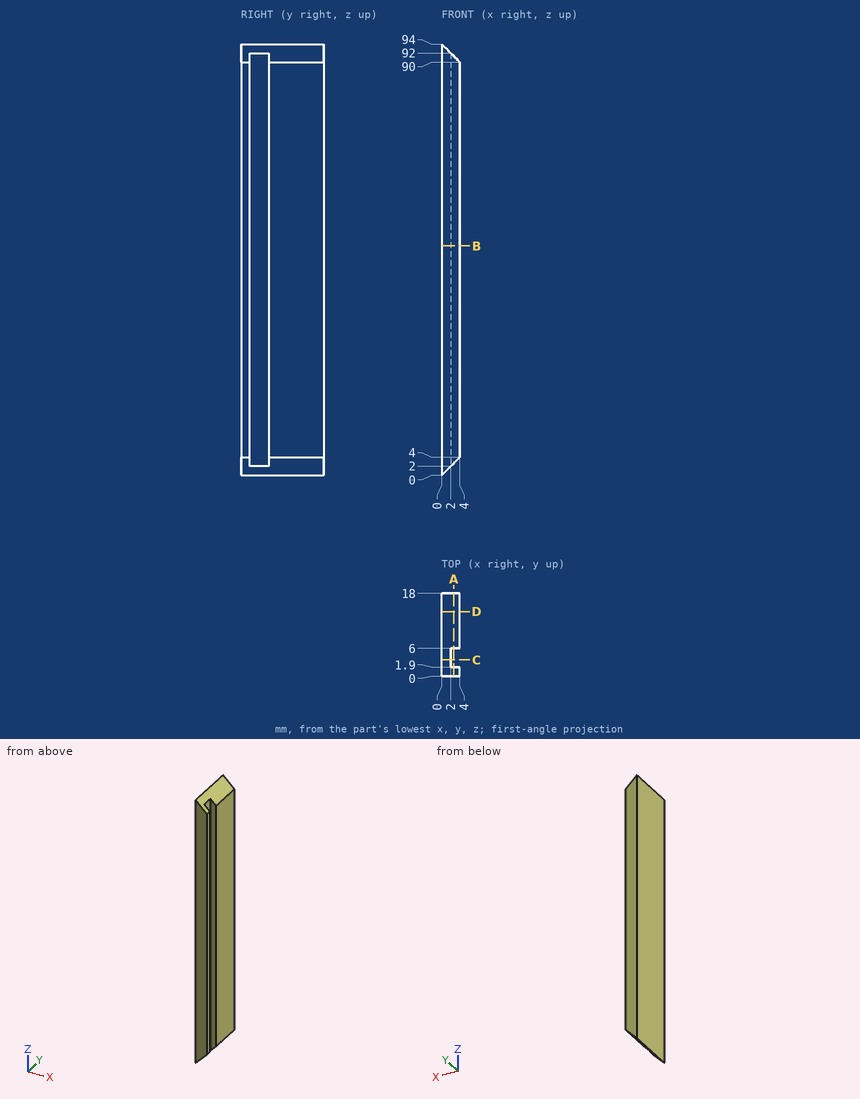
Drawing for the job (mm, zero at the part's lowest x, y, z). Round coordinates to 2 decimals unless told otherwise and drop trailing zeros. Order: outer loops, then holes, each group sorted by start corner. A loop starts at its lowest first (then second) coordinate and runs counter-clockwise, first axis right, second up. Notation, with made-up numbers: (-33.5, -32) -> (2.5, -32) arc R26 ccw to (2.5, -15) -> close; hole circle Ø9 at (85, 54). An arc over 180 degrees is marked (long way). Write item = value, one per line. Start each with the question number.
(1) Probe line 1 (Y direction, x = 2.5, z = 50); line 2 (X direction, y = 3.25, z = 63); line 3 (Z direction, x = 0.2, y = 13.75). List the from-to ranges inside material, lowest first. Write a range as [from, to].
(2) Cut at B-B, the plane z = 50. List the corners of the cut face in (x, y).
(3) Cut at A-A, the plane x = 2.65. List the corners of the cut face in (y, z).
(4) Cut at D-D, the plane y = 14. List the corners of the cut face in (x, z).
(5) Pin check, flat tip, straight feed: P1, Ø1.5, axis at x = 1.5, y = 10.5, coming from the +Z side. Stop position of the tip, or through.
(6) Cut at C-C, the plane y = 3.5. List the corners of the cut face in (x, z), then the cut area to 3 significant figures.
Model answer:
q1.line_1 = [0, 1.9], [6, 18]
q1.line_2 = [0, 2]
q1.line_3 = [0.2, 93.8]
q2.outline = (0, 0) -> (4, 0) -> (4, 1.9) -> (2, 1.9) -> (2, 6) -> (4, 6) -> (4, 18) -> (0, 18) -> close
q3.outline = (0, 2.65) -> (1.9, 2.65) -> (1.9, 91.35) -> (0, 91.35) -> close; (6, 2.65) -> (18, 2.65) -> (18, 91.35) -> (6, 91.35) -> close
q4.outline = (0, 0) -> (4, 4) -> (4, 90) -> (0, 94) -> close
q5.P1 = 93.25
q6.outline = (0, 0) -> (2, 2) -> (2, 92) -> (0, 94) -> close
q6.area = 184 mm2
